The drawing under review shows one solid part. Ordinate dimensions are in mm from its lowest x, y, z. A direction names the side the tool comes from. Round coordinates to 2 decimals unless told otherwise and drop trailing zeros. Loops run counter-clockwise (first coordinate to the right, second up) from the corner with the lowest first, then second, coordinate; pieces in that order, holes last. Notation, with made-up numbers: M 23,-14 L 79,-14 A7 ccw 79,-2 Z; hole C -9.75,-15.5 d1. An arc over 180 degrees is marked long. Use a Markdown table: item, result.
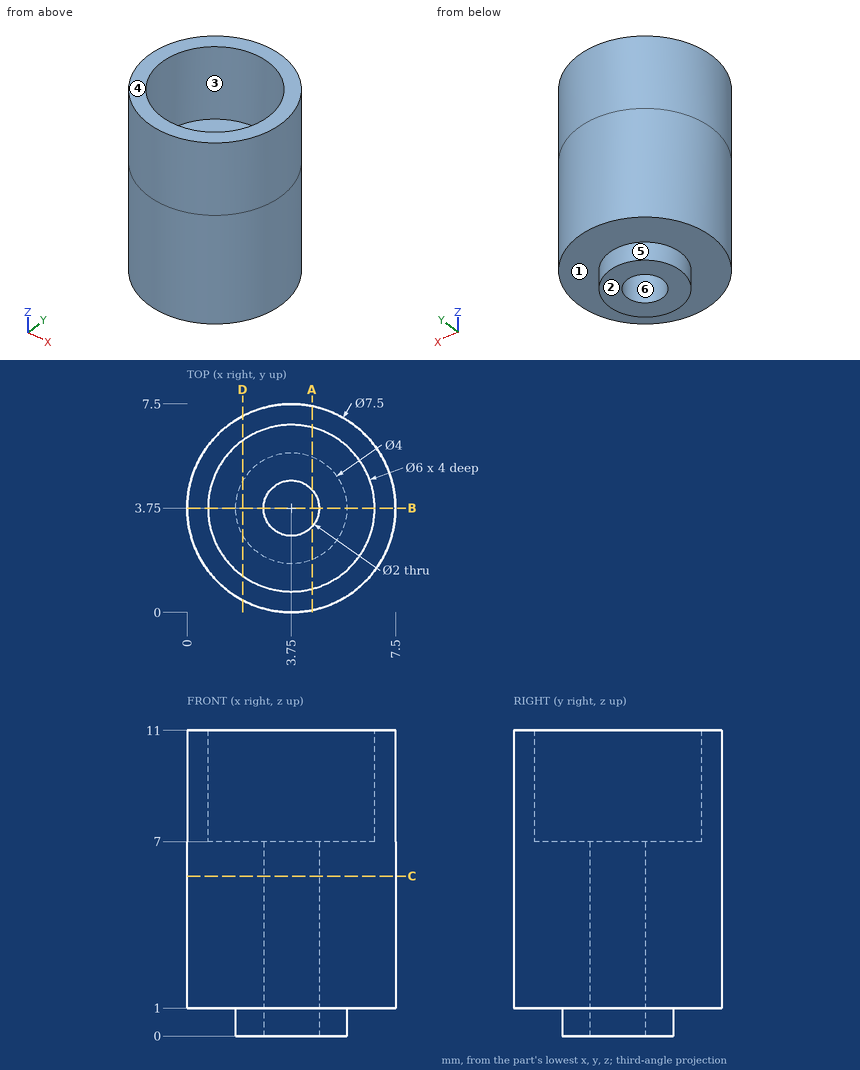
1. Take a section at A-A on x = 4.5. Give the boundary of the cut face in (y, z).
Check values:
| item | result |
|---|---|
| outline | M 0.08,1 L 1.9,1 L 1.9,0 L 3.09,0 L 3.09,7 L 0.85,7 L 0.85,11 L 0.08,11 Z; M 4.41,0 L 5.6,0 L 5.6,1 L 7.42,1 L 7.42,11 L 6.65,11 L 6.65,7 L 4.41,7 Z |
2. Take a section at C-C on z = 5.75. Give the boundary of the cut face in (x, y), and give its area (3 significant figures).
Check values:
| item | result |
|---|---|
| outline | C 3.75,3.75 d7.5; hole C 3.75,3.75 d2 |
| area | 41.0 mm² |
3. Machinability: for the marked faces 1 and 2, which of the approach directions +Z, -Z, +X, -X, +Y, -Y give a long, thin tool a straight path to every point of the face, cutting with its end or side? Answer none if there is none.
Check values:
| item | result |
|---|---|
| face 1 | -Z |
| face 2 | -Z, +X, -X, +Y, -Y |
4. Insertion check: pin 1 (1.8 mm diameter, centred on x = 4.5, y = 3, fed in from +Z); pin 2 (3 mm diameter, centred on y = 6.5, z = 4.5, fed in from +X); pin 3 (2 mm diameter, centred on x = 1, z = 7.5, fed in from +Y). Each pin has a flat end and moves straight along its axis. Give the tip position at first contact, or say it passes through.
Check values:
| item | result |
|---|---|
| pin 1 | stops at z = 7 |
| pin 2 | stops at x = 7.29 |
| pin 3 | stops at y = 7.07 |
5. The part is to be moulded in two halves that separate along X. For the marked faces 3, 4, 5 and 6, say which applies: pulls with the +X half, pulls with the -X half, needs draft (parallel to the pull), parting line crosses it, or undercut.
Check values:
| item | result |
|---|---|
| face 3 | undercut |
| face 4 | needs draft |
| face 5 | parting line crosses it |
| face 6 | undercut |
6. Wall thickness on line 1 along Y through (x, z) = (3.75, 8.7); line 2 along Y through (x, z) = (3.75, 5.5); line 3 along Z through (x, y) = (5.5, 2): over which ranges is each line inside the solid? List them lowest first. Write a range as from..to.
Check values:
| item | result |
|---|---|
| line 1 | y = 0..0.75, 6.75..7.5 |
| line 2 | y = 0..2.75, 4.75..7.5 |
| line 3 | z = 1..7 |
7. Take a section at D-D on x = 2. Give the boundary of the cut face in (y, z), and give its area (3 significant figures).
Check values:
| item | result |
|---|---|
| outline | M 0.43,1 L 2.78,1 L 2.78,0 L 4.72,0 L 4.72,1 L 7.07,1 L 7.07,11 L 6.19,11 L 6.19,7 L 1.31,7 L 1.31,11 L 0.43,11 Z |
| area | 48.8 mm² |
8. Take a section at B-B on y = 3.75. Give the boundary of the cut face in (x, z), and give its area (3 significant figures).
Check values:
| item | result |
|---|---|
| outline | M 0,1 L 1.75,1 L 1.75,0 L 2.75,0 L 2.75,7 L 0.75,7 L 0.75,11 L 0,11 Z; M 4.75,0 L 5.75,0 L 5.75,1 L 7.5,1 L 7.5,11 L 6.75,11 L 6.75,7 L 4.75,7 Z |
| area | 41.0 mm² |
